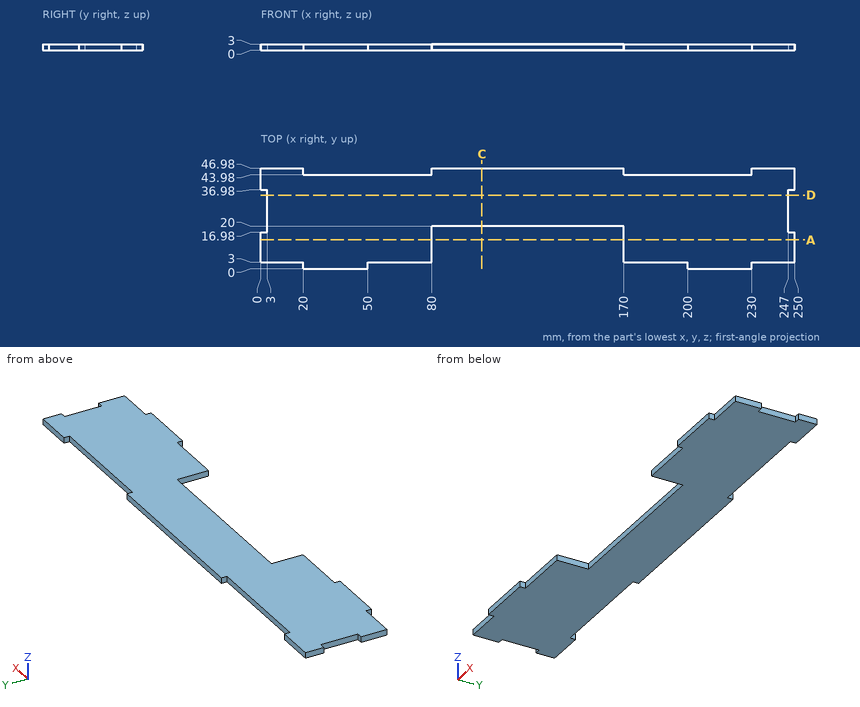
The figure shows three views and two pictorial views of one solid part (mm, origin at its lowest corner). Answer the questions. Round coordinates to 2 decimals unless told otherwise and drop trailing zeros. Order: outer loops, then holes, each group sorted by start corner. A loop starts at its lowest first (then second) coordinate and runs counter-clockwise, first axis right, second up.
Q1. A cutting plane is placed at A-A, the plane y = 13.5. Determine the outline of the cut face in (x, z).
Solution:
outline: (0, 0) - (80, 0) - (80, 3) - (0, 3) - close; (170, 0) - (250, 0) - (250, 3) - (170, 3) - close
Q2. A cutting plane is placed at C-C, the plane x = 103.5. Determine the outline of the cut face in (y, z).
Solution:
outline: (20, 0) - (46.98, 0) - (46.98, 3) - (20, 3) - close
Q3. A cutting plane is placed at D-D, the plane y = 34.5. Determine the outline of the cut face in (x, z), then the cut area to 3 significant figures.
Solution:
outline: (3, 0) - (247, 0) - (247, 3) - (3, 3) - close
area: 732 mm2
Q4. Find the intervals of material crossed by line 1 along X through (y, z) = (44.5, 0.8); line 2 along X through (y, z) = (19.5, 2.2); line 3 along X through (y, z) = (4.5, 1.45), in increasing order.
Solution:
line 1: x = 0 to 20, 80 to 170, 230 to 250
line 2: x = 3 to 80, 170 to 247
line 3: x = 0 to 80, 170 to 250
Q5. Given pin 1 Ø1.5 at (x, z) = (70.5, 2) entering from -Y, flat-ended and moving along its own axis, determine where the tip first touches the part or whether it passes through.
Solution:
pin 1: stops at y = 3
